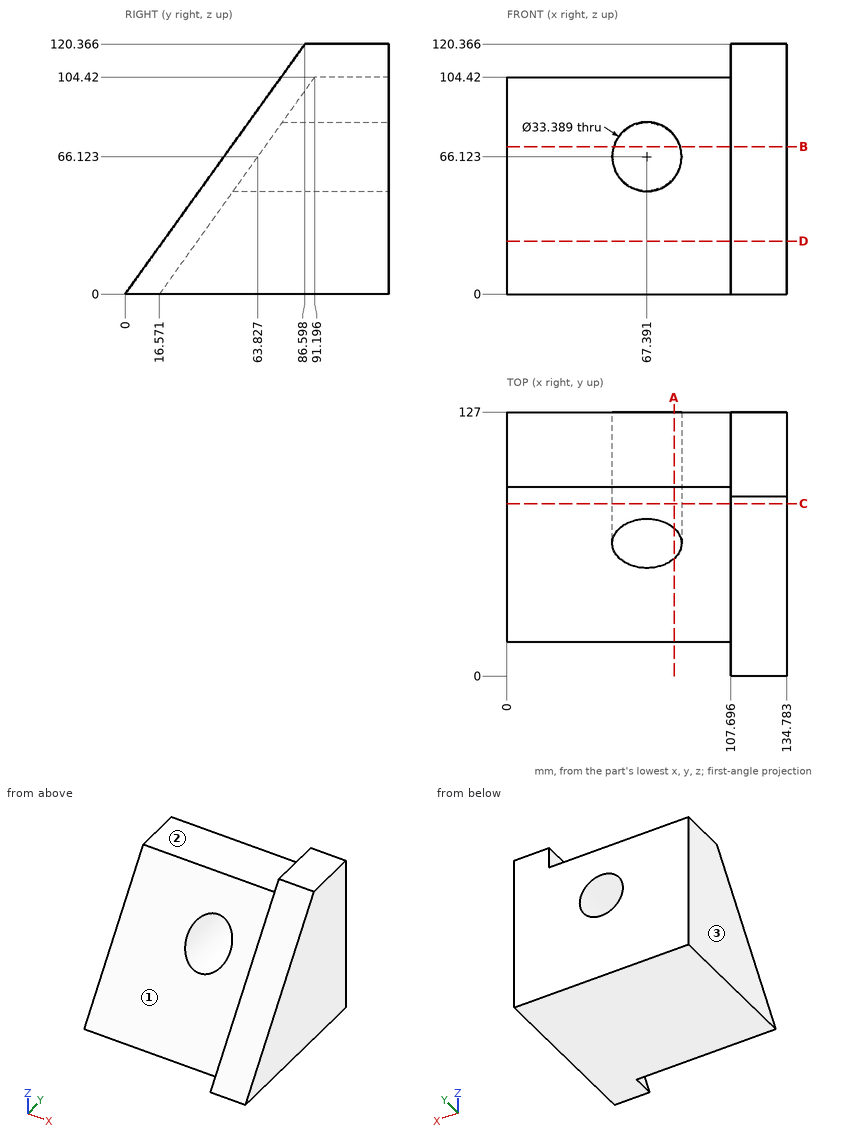
Can you work these out from the drawing? Everything is in mm from the part's minimum corner. A direction names the side the tool comes from. Round coordinates to 2 decimals unless told otherwise and drop trailing zeros. Order: outer loops, then holes, each group sorted by start corner. A loop starts at its lowest first (then second) coordinate and runs counter-clockwise, first axis right, second up. Notation, with made-up numbers: (76, 29.5) -> (116, 29.5) arc R22 cw to (116, 50.5) -> close; hole circle Ø5 at (42, -35.5). An arc over 180 degrees is marked (long way). Use CSV: the item, a comma, the result in double quotes.
1. I'm going to push flat-ended pins straight in: P1, Ø1.5, axis at x = 115, y = 22.5, coming from the +Z side (1 decimal); P2, Ø1, axis at x = 57, z = 16, coming from the -Y side; P3, Ø1.5, axis at x = 40, z = 87.5, coming from the -Y side. Where does each tip first touch, or does it pass through?
Recorded:
P1,"stops at z = 32.3"
P2,"stops at y = 27.65"
P3,"stops at y = 78.57"
2. I want a section at A-A on x = 80.5. List the corners of the cut face in (y, z) for me (1 decimal), and give its area (3 significant figures).
Recorded:
outline,"(16.6, 0) -> (127, 0) -> (127, 55.8) -> (56.4, 55.8) -> close; (71.2, 76.5) -> (127, 76.5) -> (127, 104.4) -> (91.2, 104.4) -> close"
area,"6,330 mm2"
3. I want a section at B-B on z = 71. List the corners of the cut face in (x, y) for me (1 decimal), and give its area (3 significant figures).
Recorded:
outline,"(0, 67.3) -> (51.4, 67.3) -> (51.4, 127) -> (0, 127) -> close; (83.4, 67.3) -> (107.7, 67.3) -> (107.7, 51.1) -> (134.8, 51.1) -> (134.8, 127) -> (83.4, 127) -> close"
area,"6,580 mm2"
4. Which directions (+Z, -Z, +X, -X, +Y, -Y) give clear straight access to the entire face, cutting with the end or side of a thin tool? Please do the marked faces 1, 2 and 3.
Recorded:
face 1,"+Z, -X, -Y"
face 2,"+Z, -X, +Y, -Y"
face 3,"+Z, -Z, -X, +Y, -Y"
5. I want a section at C-C on y = 83. List the corners of the cut face in (x, z) for me (1 decimal).
Recorded:
outline,"(0, 0) -> (134.8, 0) -> (134.8, 115.4) -> (107.7, 115.4) -> (107.7, 93) -> (0, 93) -> close; hole circle Ø33.4 at (67.4, 66.1)"
6. I want a section at D-D on z = 25.5. List the corners of the cut face in (x, y) for me (1 decimal), and give its area (3 significant figures).
Recorded:
outline,"(0, 34.8) -> (107.7, 34.8) -> (107.7, 18.3) -> (134.8, 18.3) -> (134.8, 127) -> (0, 127) -> close"
area,"12,900 mm2"
7. I need wall thicknesses on line 1 along Z through (x, y) = (49, 106.5); line 2 along Z through (x, y) = (59, 95) (1 decimal); line 3 along Z through (x, y) = (63.5, 78) (1 decimal). Which ranges of each line are inside material? Lowest first, please.
Recorded:
line 1,"z = 0 to 104.42"
line 2,"z = 0 to 51.7, 80.6 to 104.4"
line 3,"z = 0 to 49.9, 82.4 to 86"
